The listing builds one solid part. Answer for the finished solid, in the listing's coordinates (mm). Give positions to 0.01 mm unless a question says otherwise; leave off trailing zeros. Loops run counter-clockwise (first coordinate to the right, second up) from the corner with the lowest first, then second, coordinate; pieces in that order, holes last. Notation, with made-up numbers: (56.25, -29.75) - (97.25, -29.75) arc R18 ccw to (97.25, -8.75) - close; hole circle Ø5 at (-38.5, 46). An arc over 180 degrees is marked (long way). Answer in a Markdown table with one row per item. Add a question column.
```python
from build123d import *

# Parameters (mm, degrees)
BOSS_EXTRUDE1_DEPTH = 3
SKETCH3_R           = 15
CUT_EXTRUDE1_DEPTH  = 3
SKETCH4_R           = 0.9
CUT_EXTRUDE2_DEPTH  = 3
CIRPATTERN1_COUNT   = 5


with BuildPart() as part:
    # Sketch1 → Boss-Extrude1 (new body)
    with BuildSketch(Plane.XY):
        Polygon((-62.133450379, -27.758203286), (7.199328029, -67.670179411), (66.582879797, -14.064267615), (33.951154754, 58.977983998), (-45.599912202, 50.514666314), align=None)
    extrude(amount=BOSS_EXTRUDE1_DEPTH)

    # Sketch3 → Cut-Extrude1 (cut)
    with BuildSketch(Plane.XY.offset(3)):
        Circle(SKETCH3_R)
    extrude(amount=-CUT_EXTRUDE1_DEPTH, mode=Mode.SUBTRACT)

    # Sketch4 → Cut-Extrude2 (cut)
    with BuildSketch(Plane(origin=(0, 0, 0), x_dir=(-1, 0, 0), z_dir=(0, 0, -1))):
        with Locations((47.678329741, -21.300358522)):
            Circle(SKETCH4_R)
    cut_extrude2 = extrude(amount=-CUT_EXTRUDE2_DEPTH, mode=Mode.SUBTRACT)

    # CirPattern1: Cut-Extrude2 ×5 about axis
    cirpattern1_axis = Axis((0, 0, 0), (0, 0, 1))
    for i in range(1, CIRPATTERN1_COUNT):
        add(cut_extrude2.rotate(cirpattern1_axis, i * 360 / CIRPATTERN1_COUNT), mode=Mode.SUBTRACT)


solid = part.part
```
(1) A cutting plane is placed at A-A on y = 6. Determine the outline of the cut face in (x, z), plus the area to 3 significant figures.
(2) The mould has two halves that part along X. Classify faces 1 (the face through (-53.75, 11.93, 1.48)), 2 (the face through (-14.985, 0.66, 1.521)), 3 (the face through (36.48, -41.24, 1.48)), 4 (the face through (16, -3, 0)): pulls with the +X half, pulls with the -X half, needs draft (parallel to the pull), parting line crosses it, or undercut.
(3) Given pin 1 Ø1 at (x, z) = (-43.5, 1.5) entering from -Y; pin 2 Ø18 at (x, y) = (0, 0) entering from -Z; pin 3 Ø1.5 at (x, z) = (1, 1.5) entering from +Y; pin 4 Ø1.5 at (y, z) = (-25, 1.5) entering from -X, each flat-ended and moving along its own axis, determine where each tip first touches the part or whether it passes through.
(4) A cutting plane is placed at D-D on y = -24.5. Determine the outline of the cut face in (x, z), plus the area to 3 significant figures.
(5) Find the intervals of material crossed by line 1 along X through (y, z) = (11, 1.15); line 2 along Y through (x, z) = (13, 2.85); line 3 along Y through (x, z) = (51, 0.5), in increasing order. Write a range as [from, to].
(6) A cutting plane is placed at C-C on z = 1.6. Determine the outline of the cut face in (x, y), plus the area to 3 significant figures.
(7) A cutting plane is placed at B-B on x = -13.5. Determine the outline of the cut face in (y, z).
Evaluation:
| question | item | result |
|---|---|---|
| 1 | outline | (-55, 0) - (-13.75, 0) - (-13.75, 3) - (-55, 3) - close; (13.75, 0) - (57.62, 0) - (57.62, 3) - (13.75, 3) - close |
| 1 | area | 255 mm² |
| 2 | face 1 | pulls with the -X half |
| 2 | face 2 | undercut |
| 2 | face 3 | pulls with the +X half |
| 2 | face 4 | needs draft |
| 3 | pin 1 | stops at y = -38.77 |
| 3 | pin 2 | passes through |
| 3 | pin 3 | stops at y = 55.55 |
| 3 | pin 4 | stops at x = -61.71 |
| 4 | outline | (-61.45, 0) - (55.02, 0) - (55.02, 3) - (-61.45, 3) - close |
| 4 | area | 349 mm² |
| 5 | line 1 | x = [-53.95, -10.2], [10.2, 55.39] |
| 5 | line 2 | y = [-62.43, -7.48], [7.48, 56.75] |
| 5 | line 3 | y = [-28.13, -11.69], [-9.9, 20.82] |
| 6 | outline | (-62.13, -27.76) - (7.2, -67.67) - (66.58, -14.06) - (33.95, 58.98) - (-45.6, 50.51) - close; hole circle Ø1.8 at (-47.68, -21.3); hole circle Ø1.8 at (-34.99, 38.76); hole circle Ø30 at (0, 0); hole circle Ø1.8 at (5.52, -51.93); hole circle Ø1.8 at (26.05, 45.26); hole circle Ø1.8 at (51.09, -10.79) |
| 6 | area | 10,300 mm² |
| 7 | outline | (-55.75, 0) - (-6.54, 0) - (-6.54, 3) - (-55.75, 3) - close; (6.54, 0) - (53.93, 0) - (53.93, 3) - (6.54, 3) - close |
